Work out the finished part from the listing and answer in its coordinate system (mm). Give positions to 0.01 mm unless a question says otherwise; leave off trailing zeros. Write each loop counter-clockwise with the first axis right and the second up, starting at its lowest first coordinate (ties: lowest second). Pieces come first, ordered by that corner, then holes. Notation, with made-up numbers: (61, 42) -> (67, 42) arc R23 ccw to (67, 71) -> close; hole circle Ø2 at (-6, -5). An arc over 180 degrees is marked (long way). Use a Markdown table: item, result. Add a question column.
Q1. For a pull along Y with two mould halves and no side action, classify faces 1 (the face through (26, -11, 0.5)), 2 (the face through (89.4, -22.86, 0.25)) as pulls with the +Y half, pulls with the -Y half, needs draft (parallel to the pull), parting line crosses it, or undercut.
Q2. Section B-B, the plane y = 0 is taken. Give the vertices of the cut face in (x, z).
Q3. Section C-C, the plane x = 95 is taken. Give the vertices of the cut face in (y, z).
Q4. Section A-A, the plane x = -35 is taken. Give the vertices of the cut face in (y, z).
Q5. Section D-D, the plane z = 0.4 is taken. Give the vertices of the cut face in (x, y), plus the area to 3 significant figures.
Q6. Consider line 1 (Y direction, x = 95, z = 0.3); line 2 (Y direction, x = 0, z = 0.2); line 3 (Y direction, x = 48, z = 0.35). Determine where each line is inside the solid, lowest interval first.
from build123d import *

# Parameters (mm, degrees)
SKETCH_W        = 178
SKETCH_H        = 144
SKETCH_R        = 22
PAD_DEPTH       = 0.5
SKETCH001_R     = 2.2
POCKET_DEPTH    = 0.501
SKETCH002_R     = 7.6
POCKET001_DEPTH = 0.501


with BuildPart() as part:
    # Sketch → Pad (new body)
    with BuildSketch(Plane.XY):
        with Locations((27, -12)):
            Rectangle(SKETCH_W, SKETCH_H)
        Circle(SKETCH_R, mode=Mode.SUBTRACT)
    extrude(amount=PAD_DEPTH)

    # Sketch001 (on Face7 of Pad) → Pocket (cut, through all)
    with BuildSketch(Plane.XY.offset(0.5)):
        with Locations((-35, 48)):
            Circle(SKETCH001_R)
        with Locations((50, -72)):
            Circle(SKETCH001_R)
    extrude(amount=-POCKET_DEPTH, mode=Mode.SUBTRACT)

    # Sketch002 (on Face5 of Pocket) → Pocket001 (cut, through all)
    with BuildSketch(Plane.XY.offset(0.5)):
        with Locations((95, 12)):
            Circle(SKETCH002_R)
        with Locations((95, -28)):
            Circle(SKETCH002_R)
    extrude(amount=-POCKET001_DEPTH, mode=Mode.SUBTRACT)


solid = part.part
Result set:
| question | item | result |
|---|---|---|
| 1 | face 1 | needs draft |
| 1 | face 2 | undercut |
| 2 | outline | (-62, 0) -> (-22, 0) -> (-22, 0.5) -> (-62, 0.5) -> close; (22, 0) -> (116, 0) -> (116, 0.5) -> (22, 0.5) -> close |
| 3 | outline | (-84, 0) -> (-35.6, 0) -> (-35.6, 0.5) -> (-84, 0.5) -> close; (-20.4, 0) -> (4.4, 0) -> (4.4, 0.5) -> (-20.4, 0.5) -> close; (19.6, 0) -> (60, 0) -> (60, 0.5) -> (19.6, 0.5) -> close |
| 4 | outline | (-84, 0) -> (45.8, 0) -> (45.8, 0.5) -> (-84, 0.5) -> close; (50.2, 0) -> (60, 0) -> (60, 0.5) -> (50.2, 0.5) -> close |
| 5 | outline | (-62, -84) -> (116, -84) -> (116, 60) -> (-62, 60) -> close; hole circle Ø4.4 at (-35, 48); hole circle Ø44 at (0, 0); hole circle Ø4.4 at (50, -72); hole circle Ø15.2 at (95, -28); hole circle Ø15.2 at (95, 12) |
| 5 | area | 23,700 mm2 |
| 6 | line 1 | y = -84 to -35.6, -20.4 to 4.4, 19.6 to 60 |
| 6 | line 2 | y = -84 to -22, 22 to 60 |
| 6 | line 3 | y = -84 to -72.92, -71.08 to 60 |
